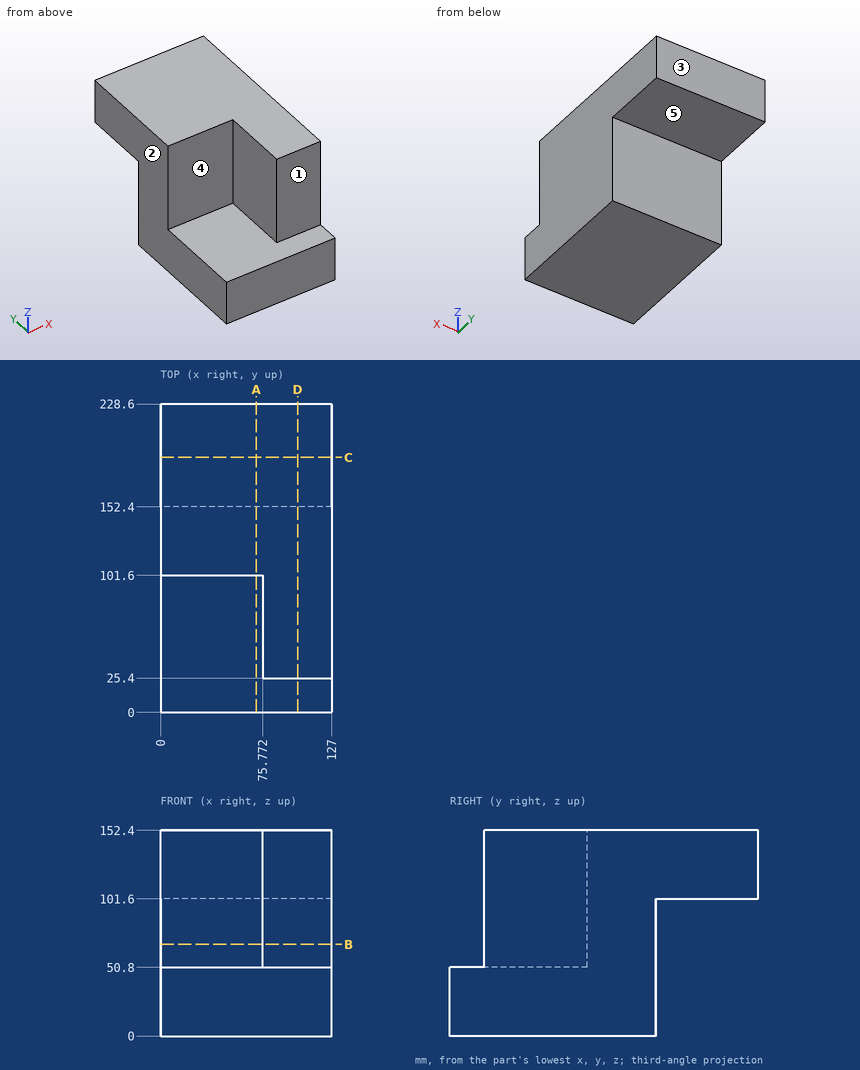
Geometry check sheet. Reference: drawing and pictorial views, mm from the part's lowest x, y, z. A direction names the side the tool comes from. Coordinates: 2 decimals unless noted, no trailing zeros. Order: outer loops, then holes, each group sorted by start corner. A loop starts at its lowest first (then second) coordinate and runs counter-clockwise, first axis right, second up. Notation, with made-up numbers: (2.25, -24) -> (54.25, -24) arc R15 cw to (54.25, -17) -> close; hole circle Ø7 at (33, -37.5). An arc over 180 degrees is marked (long way). Use CSV: the item, a comma, the result in double quotes. Start each with the question number.
Q1. Depth check by flat-ended pin: P1, Ø22.5, axis at x = 48.5, z = 104, coming from the -Y side; P2, Ø1.5, axis at x = 66, z = 49.5, coming from the +Y side. Enter the tip coordinate at first touch or a pass-through.
Q2. Section check D-D, the plane x = 101.5. Record the cut outline in (y, z).
Q3. Thickness scan on line 1 along Y through (x, z) = (55.5, 128); line 2 along Z through (x, y) = (72.5, 194.5); line 3 along Z through (x, y) = (122, 21). Record the ranges inside material, lowest first.
Q4. Section check C-C, the plane y = 189. Record the cut outline in (x, z).
Q5. Tool access check on the marked faces 1, 2, 3, 4 and 5. Record the directions out of +Z, -Z, +X, -X, +Y, -Y that give a thin tool (end or side, any length) a straight path to the whole face; none if there is none.
Q6. Section check A-A, the plane x = 71. Record the cut outline in (y, z).
Q7. Section check B-B, the plane z = 68. Record the cut outline in (x, y).
Returned:
1,P1,"stops at y = 101.6"
1,P2,"stops at y = 152.4"
2,outline,"(0, 0) -> (152.4, 0) -> (152.4, 101.6) -> (228.6, 101.6) -> (228.6, 152.4) -> (25.4, 152.4) -> (25.4, 50.8) -> (0, 50.8) -> close"
3,line 1,"y = 101.6 to 228.6"
3,line 2,"z = 101.6 to 152.4"
3,line 3,"z = 0 to 50.8"
4,outline,"(0, 101.6) -> (127, 101.6) -> (127, 152.4) -> (0, 152.4) -> close"
5,face 1,"+Z, +X, -X, -Y"
5,face 2,"+Z, -Z, -X, +Y, -Y"
5,face 3,"+Z, -Z, +X, -X, +Y"
5,face 4,"+Z, -X, -Y"
5,face 5,"-Z, +X, -X, +Y"
6,outline,"(0, 0) -> (152.4, 0) -> (152.4, 101.6) -> (228.6, 101.6) -> (228.6, 152.4) -> (101.6, 152.4) -> (101.6, 50.8) -> (0, 50.8) -> close"
7,outline,"(0, 101.6) -> (75.77, 101.6) -> (75.77, 25.4) -> (127, 25.4) -> (127, 152.4) -> (0, 152.4) -> close"
